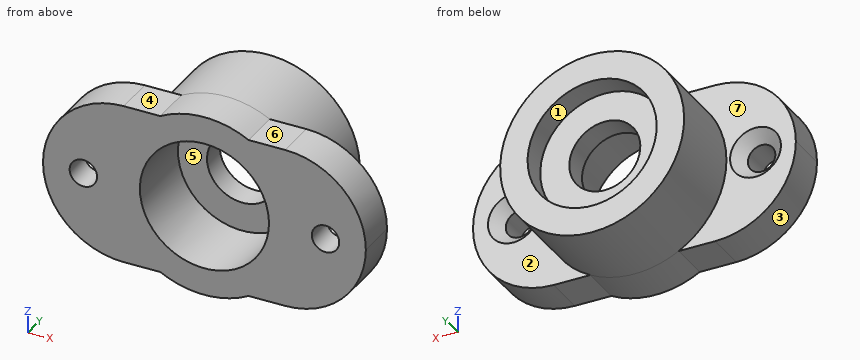
from build123d import *
from build123d.topology import SkipClean

# Parameters (mm, degrees)
SKETCH1_W                                       = 40
SKETCH1_H                                       = 20
BOSS_EXTRUDE1_DEPTH                             = 5
CSK_FOR_M3_FLAT_HEAD_MACHINE_SCREW1_D           = 3.4
CSK_FOR_M3_FLAT_HEAD_MACHINE_SCREW1_CSINK_D     = 6.3
CSK_FOR_M3_FLAT_HEAD_MACHINE_SCREW1_CSINK_ANGLE = 90
SKETCH4_R                                       = 4.4
CUT_EXTRUDE1_DEPTH                              = 5
BOSS_EXTRUDE2_START                             = 10
SKETCH5_R                                       = 11.4
SKETCH5_R_2                                     = 4.4
BOSS_EXTRUDE2_DEPTH                             = 10
FILLET1_R                                       = 10
SKETCH6_R                                       = 8
SKETCH6_R_2                                     = 4.4
CUT_EXTRUDE2_DEPTH                              = 3
CUT_EXTRUDE3_START                              = -9
SKETCH7_R                                       = 8
CUT_EXTRUDE3_DEPTH                              = 9
BOSS_EXTRUDE3_START                             = -5
BOSS_EXTRUDE3_DEPTH                             = 5


with BuildPart() as part:
    # Sketch1 → Boss-Extrude1 (new body)
    with BuildSketch(Plane(origin=(0, 0, 0), x_dir=(1, 0, 0), z_dir=(0, 1, 0))):
        Rectangle(SKETCH1_W, SKETCH1_H)
    extrude(amount=BOSS_EXTRUDE1_DEPTH)

    # CSK for M3 Flat Head Machine Screw1 (through all)
    with Locations(Plane(origin=(0, 5, 0), x_dir=(1, 0, 0), z_dir=(0, 1, 0))):
        with Locations((15, 0), (-15, 0)):
            CounterSinkHole(CSK_FOR_M3_FLAT_HEAD_MACHINE_SCREW1_D / 2, CSK_FOR_M3_FLAT_HEAD_MACHINE_SCREW1_CSINK_D / 2, counter_sink_angle=CSK_FOR_M3_FLAT_HEAD_MACHINE_SCREW1_CSINK_ANGLE)

    # Sketch4 → Cut-Extrude1 (cut)
    with BuildSketch(Plane(origin=(0, 5, 0), x_dir=(1, 0, 0), z_dir=(0, 1, 0))):
        with Locations(Location((0, 0, 0), (0, 0, 270))):
            Circle(SKETCH4_R)
    extrude(amount=-CUT_EXTRUDE1_DEPTH, mode=Mode.SUBTRACT)

    # Sketch5 → Boss-Extrude2 (add)
    with BuildSketch(Plane(origin=(0, 5, 0), x_dir=(1, 0, 0), z_dir=(0, 1, 0)).offset(BOSS_EXTRUDE2_START)):
        with Locations(Location((0, 0, 0), (0, 0, 61.305586473))):
            Circle(SKETCH5_R)
        with Locations(Location((0, 0, 0), (0, 0, 270))):
            Circle(SKETCH5_R_2, mode=Mode.SUBTRACT)
    extrude(amount=-BOSS_EXTRUDE2_DEPTH)

    # Fillet1
    fillet1_edges = [part.edges().sort_by_distance(p)[0] for p in [
        (20, 2.5, 10),
        (-20, 2.5, -10),
        (20, 2.5, -10),
        (-20, 2.5, 10),
    ]]
    fillet(fillet1_edges, radius=FILLET1_R - 0.0001)  # a hair under: the kernel refuses the full size

    # Sketch6 → Cut-Extrude2 (cut)
    with BuildSketch(Plane(origin=(0, 15, 0), x_dir=(1, 0, 0), z_dir=(0, 1, 0))):
        with Locations(Location((0, 0, 0), (0, 0, 270))):
            Circle(SKETCH6_R)
        with Locations(Location((0, 0, 0), (0, 0, 270))):
            Circle(SKETCH6_R_2, mode=Mode.SUBTRACT)
    extrude(amount=-CUT_EXTRUDE2_DEPTH, mode=Mode.SUBTRACT)

    # Sketch7 → Cut-Extrude3 (cut)
    with BuildSketch(Plane.XZ.offset(CUT_EXTRUDE3_START)):
        with Locations(Location((0, 0, 0), (0, 0, 90))):
            Circle(SKETCH7_R)
    extrude(amount=CUT_EXTRUDE3_DEPTH, mode=Mode.SUBTRACT)

    # Sketch8 → Boss-Extrude3 (add)
    with SkipClean():  # the faces are left unmerged after this step: merging them gives an invalid solid
        with BuildSketch(Plane.XZ.offset(BOSS_EXTRUDE3_START)):
            with BuildLine():
                Line((-5.473572873, 10), (5.473572873, 10))
                ThreePointArc((5.473572873, 10), (0, 11.4), (-5.473572873, 10))
            make_face()
            with BuildLine():
                Line((-5.473572873, -10), (5.473572873, -10))
                ThreePointArc((5.473572873, -10), (0, -11.4), (-5.473572873, -10))
            make_face()
        extrude(amount=BOSS_EXTRUDE3_DEPTH)


solid = part.part
The model under review builds one solid part; all positions refer to its coordinate system, in mm. Face numbers are marked on the shaded views. A direction names the side the tool comes from. Give positions to 0.01 mm unless a question says otherwise; leave off trailing zeros. Order: outer loops, then holes, each group sorted by start corner. A loop starts at its lowest first (then second) coordinate and runs counter-clockwise, first axis right, second up. Notation, with made-up numbers: M 22.5,-7.75 L 58.5,-7.75 A19 cw 58.5,20.25 Z; hole C -14.75,14.25 d6. An arc over 180 degrees is marked long. Use one line per item in the form item = value. Start each with the question number.
Item 1: The part is to be moulded in two halves that separate along X. For the marked faces 1, 2 and 3, say which applies: pulls with the +X half, pulls with the -X half, needs draft (parallel to the pull), parting line crosses it, or undercut.
Item 2: We need section A-A on y = 4.5. Give the number of separate pieces and of enclosed holes in the cut face, plus the area to 3 significant figures.
Item 3: For the marked faces 4, 5, 6 and 7, list the 3-axis set-ups (+Z, -Z, +X, -X, +Y, -Y) from which the entire face can be reached by the end or side of a thin tool; tool diameter is ignored.
Item 4: We need section B-B on x = 0. Give the boundary of the cut face in (y, z).
Item 5: We need section D-D on y = 9.5. Give the boundary of the cut face in (x, z).
Item 6: To check wall thickness, follow line 1 along X through (y, z) = (4.5, -0.5); line 2 along X through (y, z) = (5.25, 0); line 3 along Z through (x, y) = (-16.5, 1.5). State the ranges of each line that lie inside material, in increasing order. Write a range as from..to.
Item 7: We need section C-C on z = 8.5. Give the boundary of the cut face in (x, y).
Item 8: Insertion check: pin 1 Ø6 at (y, z) = (5, 1.5) entering from -X; pin 2 Ø5 at (x, y) = (-8.5, 1.5) entering from +Z; pin 3 Ø13 at (x, z) = (-0.5, -0.5) entering from +Y; pin 4 Ø6 at (y, z) = (2, 7) entering from +X. Each pin has a flat end and moves straight along its axis. Give the tip position at first contact, or say it passes through.
Completed:
q1.face_1 = undercut
q1.face_2 = needs draft
q1.face_3 = pulls with the -X half
q2.separate_pieces = 1
q2.enclosed_holes = 3
q2.area = 490 mm²
q3.face_4 = +Z, -X, +Y, -Y
q3.face_5 = -Y
q3.face_6 = +Z, +X, +Y, -Y
q3.face_7 = -X, +Y
q4.outline = M 0,-11.4 L 15,-11.4 L 15,-8 L 12,-8 L 12,-4.4 L 9,-4.4 L 9,-8 L 0,-8 Z; M 0,8 L 9,8 L 9,4.4 L 12,4.4 L 12,8 L 15,8 L 15,11.4 L 0,11.4 Z
q5.outline = C 0,0 d22.8; hole C 0,0 d8.8
q6.line_1 = -19.99..-17.6, -12.4..-7.98, 7.98..12.4, 17.6..19.99
q6.line_2 = -11.4..-8, 8..11.4
q6.line_3 = -7.6..-0.8, 0.8..7.6
q7.outline = M -15.27,0 L 15.27,0 L 15.27,5 L 7.6,5 L 7.6,15 L -7.6,15 L -7.6,5 L -15.27,5 Z
q8.pin_1 = -20
q8.pin_2 = 10
q8.pin_3 = 12
q8.pin_4 = 19.17
